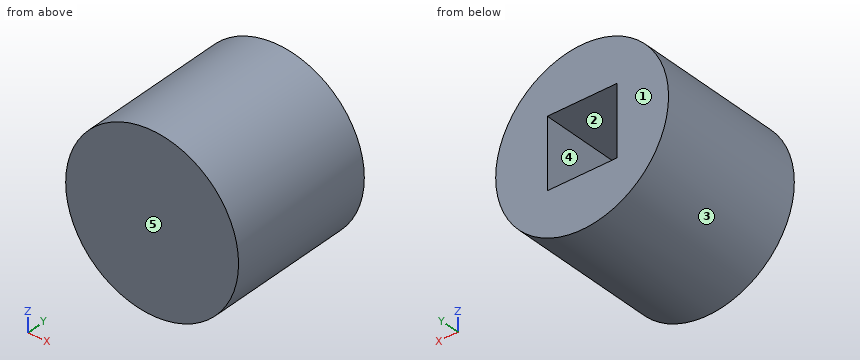
Autodesk Inventor part; units mm, degrees
ref_plane "YZ Plane" through (0, 0, 0) normal (1, 0, 0) x (0, 1, 0)
ref_plane "XZ Plane" through (0, 0, 0) normal (0, 1, 0) x (-1, 0, 0)
ref_plane "XY Plane" through (0, 0, 0) normal (0, 0, 1) x (1, 0, 0)
sketch "Sketch1" plane through (0, 0, 0) normal (0, 1, 0) x (-1, 0, 0)
  circle A0 centre (0, 0) radius 4
  dimension "d0" = 8
extrude "Extrusion1" add sketch "Sketch1" along normal blind 7
sketch "Sketch2" plane through (0, 7, 0) normal (0, 1, 0) x (1, 0, 0)
  line L0 (-1.61, -1.61) -> (1.61, -1.61)
  line L1 (1.61, -1.61) -> (1.61, 1.61)
  line L2 (1.61, 1.61) -> (-1.61, 1.61)
  line L3 (-1.61, 1.61) -> (-1.61, -1.61)
  point P0 (0, 0)
  dimension "d3" = 3.22
  dimension "d4" = 1.61
  dimension "d6" = 1.61
extrude "Extrusion2" cut sketch "Sketch2" against normal blind 5
properties part number "Wheel_cap_extended"
Geometry: final body of the model. Coordinates: model frame, mm. Face numbers are marked on the shaded views. A direction names the side the tool comes from. Give positions to 0.01 mm unless a question says otherwise; leave off trailing zeros. Order: outer loops, then holes, each group sorted by start corner. A loop starts at its lowest first (then second) coordinate and runs counter-clockwise, first axis right, second up. Notation, with made-up numbers: (37.5, 2.25) -> (75.5, 2.25) arc R18 ccw to (75.5, 26.25) -> close; hole circle Ø4 at (-35, 57.5). An arc over 180 degrees is marked (long way). Write each question's results on one line, items separated by ' | '. Start each with the question number.
1) Section A-A (z = 0). Return loops of the section in (x, y).
2) Draft query along X for the marked faces 1, 2 and 3. Return one class per face: pulls with the +X half, pulls with the -X half, needs draft (parallel to the pull), parting line crosses it, or undercut.
3) Set-up query: the marked faces 4 and 5. Return all of +Z, -Z, +X, -X, +Y, -Y with unobstructed straight access to the full face (end or side cutting, diameter ignored); none if empty.
4) Line query: line 1 (Y direction, x = -0.5, z = 0.5); line 2 (Z direction, x = -0.75, y = 5.75); line 3 (Z direction, x = 0.5, y = 6.75). Output: solid intervals per line, ascending. Write a range as from..to.
5) First-contact query: pin 1 (1.5 mm diameter, centred on x = 1, y = 1, fed in from -Z); pin 2 (1 mm diameter, centred on y = 4.5, z = -2, fed in from +X). Flat tips, straight axial feed; report the tip coordinate or a pass-through.
6) Section B-B (y = 4). Return loops of the section in (x, z).
7) Section D-D (z = -2.25). Return loops of the section in (x, y), then the cut area to 3 significant figures.
8) Section C-C (x = 0). Return loops of the section in (y, z), then the cut area to 3 significant figures.
Calculated:
1) outline: (-4, 0) -> (4, 0) -> (4, 7) -> (1.61, 7) -> (1.61, 2) -> (-1.61, 2) -> (-1.61, 7) -> (-4, 7) -> close
2) face 1: needs draft | face 2: undercut | face 3: parting line crosses it
3) face 4: +Y | face 5: +Z, -Z, +X, -X, -Y
4) line 1: 0..2 | line 2: -3.93..-1.61, 1.61..3.93 | line 3: -3.97..-1.61, 1.61..3.97
5) pin 1: z = -3.99 | pin 2: x = 3.71
6) outline: circle Ø8 at (0, 0); hole (-1.61, -1.61) -> (1.61, -1.61) -> (1.61, 1.61) -> (-1.61, 1.61) -> close
7) outline: (-3.31, 0) -> (3.31, 0) -> (3.31, 7) -> (-3.31, 7) -> close | area: 46.3 mm2
8) outline: (0, -4) -> (7, -4) -> (7, -1.61) -> (2, -1.61) -> (2, 1.61) -> (7, 1.61) -> (7, 4) -> (0, 4) -> close | area: 39.9 mm2
